Input: dimensioned drawing with shaded views. Units: mm. Origin: part minimum x, y, z. Round coordinates to 2 decimals unless told otherwise and drop trailing zeros. Loops run counter-clockwise (first coordinate to the right, second up) from the corner with the lowest first, then second, coordinate; pieces in that order, holes last. Notation, with made-up numbers: (15, -26.75) - (69, -26.75) arc R18 cw to (69, -8.75) - close; hole circle Ø1 at (72, -32.75). An arc over 180 degrees is marked (long way). Write each question's results on one line, items separated by ' | '.
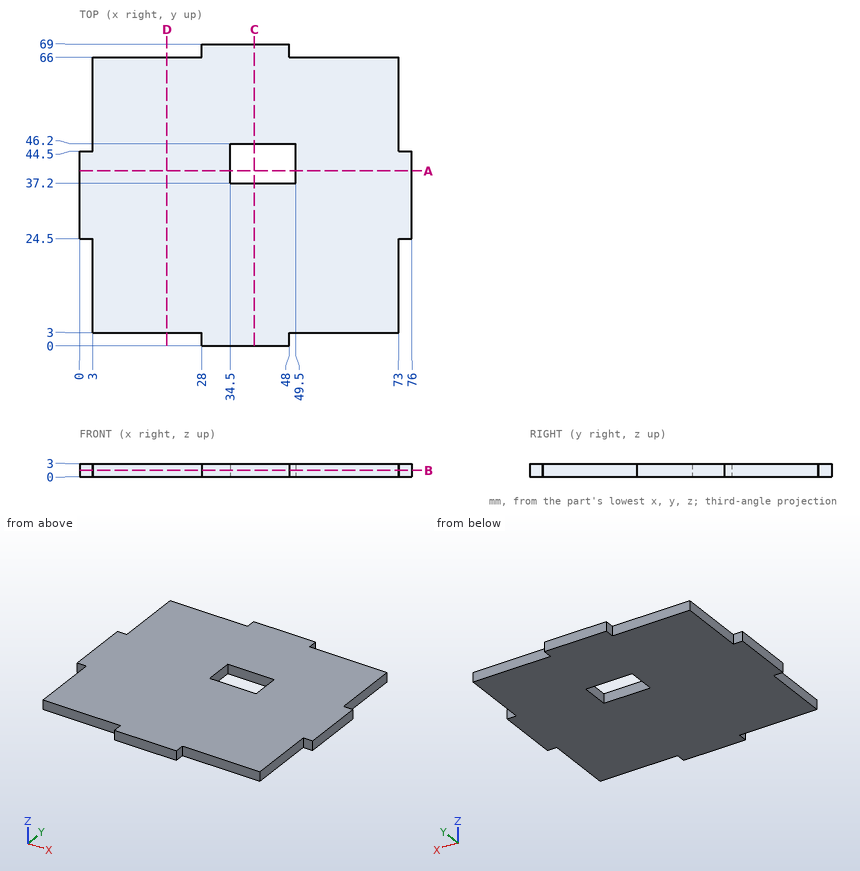
1. Line query: line 1 (Y direction, x = 38, z = 1.1); line 2 (X direction, y = 45, z = 0.5); line 3 (Y direction, x = 48.5, z = 2.65). Output: solid intervals per line, ascending. Write a range as [from, to].
Answer:
line 1: [0, 37.2], [46.2, 69] | line 2: [3, 34.5], [49.5, 73] | line 3: [3, 37.2], [46.2, 66]
2. Section query C-C, the plane x = 40. Output: boundary loops of the cut face in (y, z), plus the area to 3 significant figures.
Answer:
outline: (0, 0) - (37.2, 0) - (37.2, 3) - (0, 3) - close; (46.2, 0) - (69, 0) - (69, 3) - (46.2, 3) - close | area: 180 mm^2
3. Section query D-D, the plane x = 20. Output: boundary loops of the cut face in (y, z), plus the area to 3 significant figures.
Answer:
outline: (3, 0) - (66, 0) - (66, 3) - (3, 3) - close | area: 189 mm^2
4. Section query B-B, the plane z = 1.5. Output: boundary loops of the cut face in (x, y), plus the area to 4 significant figures.
Answer:
outline: (0, 24.5) - (3, 24.5) - (3, 3) - (28, 3) - (28, 0) - (48, 0) - (48, 3) - (73, 3) - (73, 24.5) - (76, 24.5) - (76, 44.5) - (73, 44.5) - (73, 66) - (48, 66) - (48, 69) - (28, 69) - (28, 66) - (3, 66) - (3, 44.5) - (0, 44.5) - close; hole (34.5, 37.2) - (49.5, 37.2) - (49.5, 46.2) - (34.5, 46.2) - close | area: 4,515 mm^2
5. Contact query for flat-ended pins moving along their axis: pin 1 (1.5 mm diameter, centred on x = 17.5, z = 1.5, fed in from +Y); pin 2 (0.9 mm diameter, centred on x = 45, z = 2, fed in from -Y); pin 3 (1.5 mm diameter, centred on y = 51, z = 2, fed in from +X); pin 4 (1.5 mm diameter, centred on x = 74, z = 2, fed in from -Y). Output: stop coordinate, or through.
Answer:
pin 1: y = 66 | pin 2: y = 0 | pin 3: x = 73 | pin 4: y = 24.5
6. Section query A-A, the plane y = 40. Output: boundary loops of the cut face in (x, z).
Answer:
outline: (0, 0) - (34.5, 0) - (34.5, 3) - (0, 3) - close; (49.5, 0) - (76, 0) - (76, 3) - (49.5, 3) - close
